Geometry: final body of the model. Coordinates: model frame, mm. A direction names the side the tool comes from. Coordinates: 2 decimals unless noted, no trailing zeros. Order: outer loops, then holes, each group sorted by start corner. A loop starts at its lowest first (then second) coordinate and runs counter-clockwise, first axis right, second up. Notation, with made-up numbers: (69.5, -18) - (104.5, -18) arc R24 ccw to (104.5, -2) - close; hole circle Ø5 at (49.25, -27). An arc over 180 degrees is marked (long way). Use one line per item in the form item = value. Start each with the question number.
```python
from build123d import *

# Parameters (mm, degrees)
BOSS_EXTRUDE1_DEPTH              = 19.05
CUT_EXTRUDE1_DEPTH               = 159.823046871
FILLET1_R                        = 25.4
F_1_8_0_125_DIAMETER_HOLE1_D     = 3.175
F_1_8_0_125_DIAMETER_HOLE1_DEPTH = 11.1252
F_1_8_0_125_DIAMETER_HOLE1_TIP   = 0.953866233


with BuildPart() as part:
    # Sketch1 → Boss-Extrude1 (new body)
    with BuildSketch(Plane(origin=(0, 0, 0), x_dir=(1, 0, 0), z_dir=(0, 1, 0))):
        with BuildLine():
            Line((7.9375, 111.6203), (7.9375, -4.582717762))
            Line((7.9375, -4.582717762), (-90.893507667, -61.642826643))
            ThreePointArc((-90.893507667, -61.642826643), (-101.73633431, -58.7375), (-98.831007667, -47.894673357))
            Line((-98.831007667, -47.894673357), (-7.9375, 4.582717762))
            Line((-7.9375, 4.582717762), (-7.9375, 111.6203))
            ThreePointArc((-7.9375, 111.6203), (0, 119.5578), (7.9375, 111.6203))
        make_face()
    extrude(amount=BOSS_EXTRUDE1_DEPTH)

    # Sketch2 → Cut-Extrude1 (cut, through all)
    with BuildSketch(Plane(origin=(0, 19.05, 0), x_dir=(1, 0, 0), z_dir=(0, 1, 0))):
        with BuildLine():
            Line((-90.893507667, -61.642826643), (-84.931832215, -58.200851716))
            ThreePointArc((-84.931832215, -58.200851716), (-90.389422779, -51.035617044), (-98.831007667, -47.894673357))
            ThreePointArc((-98.831007667, -47.894673357), (-101.73633431, -58.7375), (-90.893507667, -61.642826643))
        make_face()
    extrude(amount=-CUT_EXTRUDE1_DEPTH, mode=Mode.SUBTRACT)

    # Fillet1
    fillet1_edges = [part.edges().sort_by_distance(p)[0] for p in [
        (7.9375, 9.525, 4.582717762),
        (-7.9375, 9.525, -4.582717762),
    ]]
    fillet(fillet1_edges, radius=FILLET1_R)

    # 1/8 (0.125) Diameter Hole1
    with Locations(Plane(origin=(0, 0, 0), x_dir=(-1, 0, 0), z_dir=(0, -1, 0))):
        with Locations((0, 94.1578), (66.903536959, -38.626775073), (3.402954744, 1.964696837)):
            Hole(F_1_8_0_125_DIAMETER_HOLE1_D / 2, depth=F_1_8_0_125_DIAMETER_HOLE1_DEPTH)
            with Locations((0, 0, -(F_1_8_0_125_DIAMETER_HOLE1_DEPTH + F_1_8_0_125_DIAMETER_HOLE1_TIP / 2))):  # 118° drill point
                Cone(0, F_1_8_0_125_DIAMETER_HOLE1_D / 2, F_1_8_0_125_DIAMETER_HOLE1_TIP, mode=Mode.SUBTRACT)


solid = part.part
```
(1) Material intervals for L1, parallel to Z at x = 0, y = 8.5; L2, parallel to X at y = 4.25, z = -23; L3, parallel to Z at x = -25.5, y = 1, sorted ascending. Write a range as from..to.
(2) Contact query for flat-ended pins moving along their axis: pin 1 Ø1 at (y, z) = (13.5, -55.5) entering from -X; pin 2 Ø4 at (y, z) = (6, 4) entering from -X; pin 3 Ø1.5 at (y, z) = (2.5, 25.5) entering from -X. Output: stop coordinate, or through.
(3) Cut plane C-C on x = -32. Return the cut outline in (y, z).
(4) Cut plane A-A on y = 7.5. Return the cut outline in (x, z) (1 decimal), plus the area to 3 significant figures.
(5) Set-up query: faces 4 (the cylindrical face through (-0.3, 5.6, -92.6)), 5 (the flat face through (7.938, 9, -62)), 6 (the flat face through (-7.938, 9, -65)). Return all of +Z, -Z, +X, -X, +Y, -Y with unobstructed straight access to the full face (end or side cutting, diameter ignored); none if empty.
(6) Cut plane B-B on z = -99. Return the cut outline in (x, y), plus the area to 3 significant figures.
(7) Draft query along Z for faces 1 (the conical face through (-66.685, 11.913, 38.795)), 2 (the flat face through (-60.282, 9.392, 25.638)), 3 (the cylindrical face through (-90.3, 9.7, 51.1)). Return one class per face: released by +Z, released by -Z, zero draft, split by the parting line, or undercut.
Check sheet entries:
q1.L1 = -119.56..-95.75, -92.57..8.36
q1.L2 = -7.94..7.94
q1.L3 = 5.56..23.89
q2.pin_1 = -7.94
q2.pin_2 = -26.27
q2.pin_3 = -61.34
q3.outline = (0, 9.31) - (19.05, 9.31) - (19.05, 27.64) - (0, 27.64) - close
q4.outline = (-98.8, 47.9) - (-20.6, 2.7) arc R25.4 cw to (-7.9, -19.2) - (-7.9, -111.6) arc R7.9 ccw to (7.9, -111.6) - (7.9, -10.1) arc R25.4 ccw to (-4.8, 11.9) - (-84.9, 58.2) arc R16.2 cw to start; hole circle Ø3.2 at (-66.9, 38.6); hole circle Ø3.2 at (-3.4, -2); hole circle Ø3.2 at (0, -94.2)
q4.area = 3,500 mm^2
q5.face_4 = -Y
q5.face_5 = +Z, -Z, +X, +Y, -Y
q5.face_6 = -Z, -X, +Y, -Y
q6.outline = (-7.94, 0) - (7.94, 0) - (7.94, 19.05) - (-7.94, 19.05) - close
q6.area = 302 mm^2
q7.face_1 = undercut
q7.face_2 = released by -Z
q7.face_3 = released by +Z
